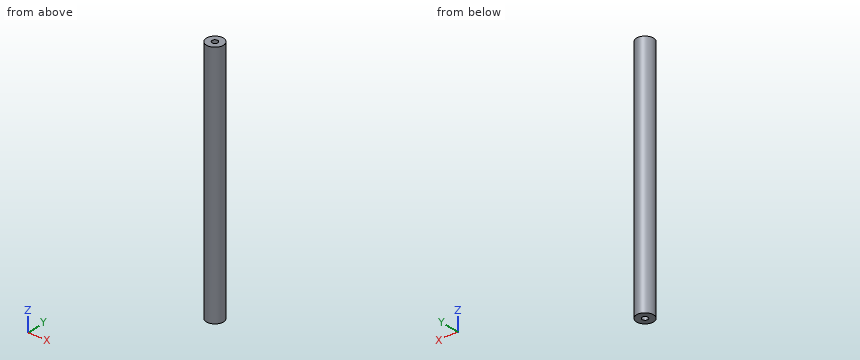
from build123d import *

# Parameters (mm, degrees)
SKETCH_1_R                        = 15
EXTRUDE_1_DEPTH                   = 217
HOLE_WIZARD_M12_1_D               = 10.2
HOLE_WIZARD_M12_1_DEPTH           = 29.25
HOLE_WIZARD_M12_1_TIP             = 3.064389157
HOLE_WIZARD_M12_1_ON_FACE_2_D     = 10.2
HOLE_WIZARD_M12_1_ON_FACE_2_DEPTH = 29.25
HOLE_WIZARD_M12_1_ON_FACE_2_TIP   = 3.064389157


with BuildPart() as part:
    # 草图1 → 凸台-拉伸1 (new body, symmetric)
    with BuildSketch(Plane.XY):
        Circle(SKETCH_1_R)
    extrude(amount=EXTRUDE_1_DEPTH, both=True)

    # M12 螺纹孔1
    with Locations(Plane.XY.offset(217)):
        with Locations((0, 0)):
            Hole(HOLE_WIZARD_M12_1_D / 2, depth=HOLE_WIZARD_M12_1_DEPTH)
            with Locations((0, 0, -(HOLE_WIZARD_M12_1_DEPTH + HOLE_WIZARD_M12_1_TIP / 2))):  # 118° drill point
                Cone(0, HOLE_WIZARD_M12_1_D / 2, HOLE_WIZARD_M12_1_TIP, mode=Mode.SUBTRACT)

    # M12 螺纹孔1 on face 2
    with Locations(Plane(origin=(0, 0, -217), x_dir=(-1, 0, 0), z_dir=(0, 0, -1))):
        with Locations((0, 0)):
            Hole(HOLE_WIZARD_M12_1_ON_FACE_2_D / 2, depth=HOLE_WIZARD_M12_1_ON_FACE_2_DEPTH)
            with Locations((0, 0, -(HOLE_WIZARD_M12_1_ON_FACE_2_DEPTH + HOLE_WIZARD_M12_1_ON_FACE_2_TIP / 2))):  # 118° drill point
                Cone(0, HOLE_WIZARD_M12_1_ON_FACE_2_D / 2, HOLE_WIZARD_M12_1_ON_FACE_2_TIP, mode=Mode.SUBTRACT)


solid = part.part
Could you check a few things on this model? Use its own coordinates, in mm. Give positions to 0.01 mm unless a question says otherwise; leave off trailing zeros. Loops run counter-clockwise (first coordinate to the right, second up) from the corner with the lowest first, then second, coordinate; pieces in that order, holes last. Notation, with made-up numbers: (76.25, -29) -> (99.25, -29) arc R15 cw to (99.25, 0) -> close; hole circle Ø1 at (-36, 66.5). An arc over 180 degrees is marked (long way). Return JSON: item names as keys, results as strings.
Item 1: If we section it at B-B on y = -10.25: List the corners of the cut face in (x, z) for me, plus the area to 3 significant figures.
Geometry results:
{"outline": "(-10.95, -217) -> (10.95, -217) -> (10.95, 217) -> (-10.95, 217) -> close", "area": "9,510 mm²"}
Item 2: If we section it at A-A on z = -43.5: List the corners of the cut face in (x, y) for me, plus the area to 3 significant figures.
Geometry results:
{"outline": "circle Ø30 at (0, 0)", "area": "707 mm²"}
Item 3: I'm going to push flat-ended pins straight in: pin 1 (5 mm diameter, centred on x = -1, y = -0.5, fed in from -Z); pin 2 (2 mm diameter, centred on x = -9.5, z = 143, fed in from -Y); pin 3 (10 mm diameter, centred on y = -7.5, z = -81, fed in from +X). Where does each tip first touch, or does it pass through?
Geometry results:
{"pin 1": "stops at z = -186.86", "pin 2": "stops at y = -12.36", "pin 3": "stops at x = 14.79"}
Item 4: I need wall thicknesses on L1, parallel to Y at x = 0, z = -203.5; L2, parallel to X at y = 0.75, z = 176; L3, parallel to Y at x = 11.5, z = -74.5. Which ranges of each line are inside material? Lowest first, please. Write a range as from..to.
Geometry results:
{"L1": "y = -15..-5.1, 5.1..15", "L2": "x = -14.98..14.98", "L3": "y = -9.63..9.63"}
